```python
from build123d import *

# Parameters (mm, degrees)
SKETCH_R     = 3.8
PAD_DEPTH    = 1.4
SKETCH001_R  = 2.3
PAD001_DEPTH = 25
SKETCH002_R  = 1.491152
PAD002_DEPTH = 1
SKETCH003_R  = 2.3
PAD003_DEPTH = 2
CHAMFER_SIZE = 0.25


with BuildPart() as part:
    # Sketch → Pad (new body)
    with BuildSketch(Plane.XY):
        Circle(SKETCH_R)
    extrude(amount=PAD_DEPTH)

    # Sketch001 (on Face3 of Pad) → Pad001 (join)
    with BuildSketch(Plane.XY.offset(1.4)):
        Circle(SKETCH001_R)
    extrude(amount=PAD001_DEPTH)

    # Sketch002 (on Face5 of Pad001) → Pad002 (join)
    with BuildSketch(Plane.XY.offset(26.4)):
        Circle(SKETCH002_R)
    extrude(amount=PAD002_DEPTH)

    # Sketch003 (on Face7 of Pad002) → Pad003 (join)
    with BuildSketch(Plane.XY.offset(27.4)):
        Circle(SKETCH003_R)
    extrude(amount=PAD003_DEPTH)

    # Chamfer
    chamfer_edges = [part.edges().sort_by_distance(p)[0] for p in [
        (-2.3, 0, 29.4),
        (-3.8, 0, 0),
    ]]
    chamfer(chamfer_edges, length=CHAMFER_SIZE)


solid = part.part
```
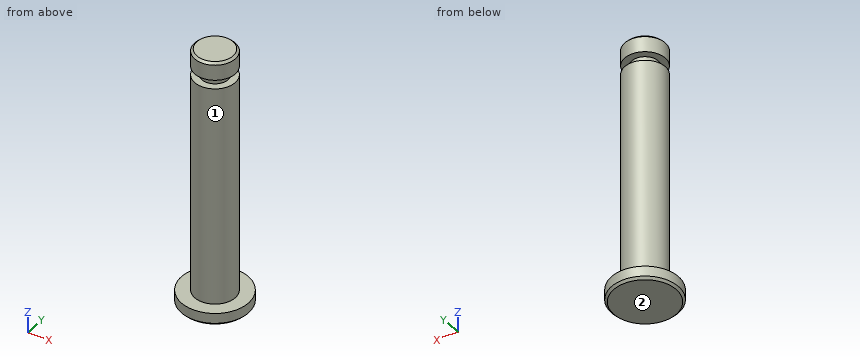
CAD build for the part. Positions are in the model's coordinates, mm. Face numbers are marked on the shaded views. A direction names the side the tool comes from. Coordinates: 2 decimals unless noted, no trailing zeros. Write each loop counter-clockwise with the first axis right and the second up, starting at its lowest first coordinate (ties: lowest second). Pieces come first, ordered by that corner, then holes. Notation, with made-up numbers: (-27.75, -12.5) -> (3.25, -12.5) arc R14 cw to (3.25, 5.5) -> close; hole circle Ø9 at (-34, 21). An arc over 180 degrees is marked (long way). Return JSON: item names as keys, results as strings. Group by question number.
Q1. Drill centre lines: line 1 (Z direction, x = 1.75, y = -1); line 2 (X direction, y = 1.75, z = 24.25); line 3 (Z direction, x = -3, y = -1.25). Where is each one in solid material? Low to high.
Q2. Cut at C-C, the plane z = 17.5. Give the cut face in (x, y).
Q3. Cut at A-A, the plane y = 0. Give the cut face in (x, z), then the cut area to 3 significant figures.
Q4. Flat gauge pins, fed straight in: pin 1 (2 mm diameter, centred on x = -2.5, y = -2.5, fed in from +Z); pin 2 (3 mm diameter, centred on y = 0, z = 16.5, fed in from +X); pin 3 (3 mm diameter, centred on x = -1, z = 25, fed in from +Y). Where does each tip first touch, or does it go through?
Q5. Which spindle directions (+Z, -Z, +X, -X, +Y, -Y) get a long thin tool onto all of the face, cutting with end or side? Do the marked faces 1 and 2. Say none if no direction does.
Returned:
{
 "1": {"line 1": "z = 0 to 26.4, 27.4 to 29.4", "line 2": "x = -1.49 to 1.49", "line 3": "z = 0 to 1.4"},
 "2": {"outline": "circle Ø4.6 at (0, 0)"},
 "3": {"outline": "(-3.8, 0.25) -> (-3.55, 0) -> (3.55, 0) -> (3.8, 0.25) -> (3.8, 1.4) -> (2.3, 1.4) -> (2.3, 26.4) -> (1.49, 26.4) -> (1.49, 27.4) -> (2.3, 27.4) -> (2.3, 29.15) -> (2.05, 29.4) -> (-2.05, 29.4) -> (-2.3, 29.15) -> (-2.3, 27.4) -> (-1.49, 27.4) -> (-1.49, 26.4) -> (-2.3, 26.4) -> (-2.3, 1.4) -> (-3.8, 1.4) -> close", "area": "138 mm2"},
 "4": {"pin 1": "stops at z = 1.4", "pin 2": "stops at x = 2.3", "pin 3": "stops at y = 2.3"},
 "5": {"face 1": "+Z", "face 2": "-Z, +X, -X, +Y, -Y"}
}
